Autodesk Inventor part; units mm, degrees
ref_plane "YZ Plane" through (0, 0, 0) normal (1, 0, 0) x (0, 1, 0)
ref_plane "XZ Plane" through (0, 0, 0) normal (0, 1, 0) x (-1, 0, 0)
ref_plane "XY Plane" through (0, 0, 0) normal (0, 0, 1) x (1, 0, 0)
sketch "Skizze1" plane through (0, 0, 0) normal (0, 0, 1) x (1, 0, 0)
  circle A0 centre (0, 0) radius 12
  circle A1 centre (0, 0) radius 2.5
  dimension "d0" = 24
  dimension "d1" = 5
extrude "Extrusion1" add sketch "Skizze1" along normal blind 2.5
sketch "Skizze2" plane through (0, 0, 0) normal (0, 0, 1) x (1, 0, 0)
  circle A0 centre (-10.4, -1.3) radius 0.75
  circle A1 centre (-10.4, 1.3) radius 0.75
  line L0 (-13.98, 0) -> (2.33, 0)
  line L1 (0, 2.87) -> (0, -2.87)
  point P0 (0, 0)
  dimension "d4" = 1.5
  dimension "d5" = 1.5
  dimension "d6" = 1.3
  dimension "d7" = 1.3
  dimension "d8" = 10.4
  dimension "d9" = 10.4
extrude "Extrusion2" cut sketch "Skizze2" along normal blind 6.75
sketch "Skizze3" plane through (0, 0, 0) normal (0, 0, -1) x (-1, 0, 0)
  circle A0 centre (0, 6) radius 1.4
  line L0 (-16.8, 0) -> (16.8, 0)
  line L1 (0, -16.8) -> (0, 16.8)
  circle A1 centre (-6, 0) radius 1.4
  circle A2 centre (0, -6) radius 1.4
  circle A3 centre (6, 0) radius 1.4
  point P0 (0, 0)
  point P1 (7.4, 0)
  point P2 (4.6, 0)
  point P3 (-4.6, 0)
  point P4 (-7.4, 0)
  point P5 (0, -4.6)
  point P6 (0, -7.4)
  point P7 (0, 4.6)
  point P8 (0, 7.4)
  dimension "d12" = 2.8
  dimension "d13" = 6
  dimension "d14" = 0
  dimension "d20" = 360
extrude "Extrusion3" cut sketch "Skizze3" against normal blind 6.75
properties part number "_3D-Druck"
Design review of the part built by this model. Coordinates are the model's own, in mm. Give positions to 0.01 mm unless a question says otherwise; leave off trailing zeros. Loops run counter-clockwise (first coordinate to the right, second up) from the corner with the lowest first, then second, coordinate; pieces in that order, holes last. Notation, with made-up numbers: M 82,-11 L 137,-11 A21 ccw 137,22 Z; hole C 86,79 d11. An arc over 180 degrees is marked long. One line per question, with ' | ' between items. Start each with the question number.
1. The part is to be moulded in two halves that separate along X. For faces 1 (the face through (-0.54, 2.44, 1.23)), 2 (the face through (0, 3, 0)), 3 (the face through (-11.99, -0.53, 1.23)), say which applies: released by +X, released by -X, zero draft, split by the parting line, or undercut.
2. To check wall thickness, follow L1, parallel to Y at x = 0, z = 1.7; L2, parallel to X at y = -1.25, z = 2.4; L3, parallel to X at y = 1, z = 1.45. State the ranges of each line that lie inside material, in increasing order.
3. Add section B-B (y = -7). Write out the cut boundary in (x, z), plus the area to 3 significant figures.
4. Add section D-D (y = -1.75). Write out the cut boundary in (x, z).
5. Add section C-C (x = 6.25). Write out the cut boundary in (y, z), plus the area to 3 significant figures.
6. Insertion check: P1, Ø1.7, axis at x = 6, y = 0, coming from the -Z side. The pin has a flat end and moves straight along its axis. Give the tip position at first contact, or say it passes through.
7. Add section A-A (z = 1.4). Write out the cut boundary in (x, y), plus the area to 3 significant figures.
Worked out:
1) face 1: undercut | face 2: zero draft | face 3: split by the parting line
2) L1: y = -12 to -7.4, -4.6 to -2.5, 2.5 to 4.6, 7.4 to 12 | L2: x = -11.93 to -11.15, -9.65 to -6.63, -5.37 to -2.17, 2.17 to 5.37, 6.63 to 11.93 | L3: x = -11.96 to -11.09, -9.71 to -6.98, -5.02 to -2.29, 2.29 to 5.02, 6.98 to 11.96
3) outline: M -9.75,0 L -0.98,0 L -0.98,2.5 L -9.75,2.5 Z; M 0.98,0 L 9.75,0 L 9.75,2.5 L 0.98,2.5 Z | area: 43.8 mm²
4) outline: M -11.87,0 L -11,0 L -11,2.5 L -11.87,2.5 Z; M -9.8,0 L -1.79,0 L -1.79,2.5 L -9.8,2.5 Z; M 1.79,0 L 11.87,0 L 11.87,2.5 L 1.79,2.5 Z
5) outline: M -10.24,0 L -1.38,0 L -1.38,2.5 L -10.24,2.5 Z; M 1.38,0 L 10.24,0 L 10.24,2.5 L 1.38,2.5 Z | area: 44.3 mm²
6) P1: passes through
7) outline: C 0,0 d24; hole C -10.4,-1.3 d1.5; hole C -10.4,1.3 d1.5; hole C -6,0 d2.8; hole C 0,0 d5; hole C 0,-6 d2.8; hole C 0,6 d2.8; hole C 6,0 d2.8 | area: 405 mm²
